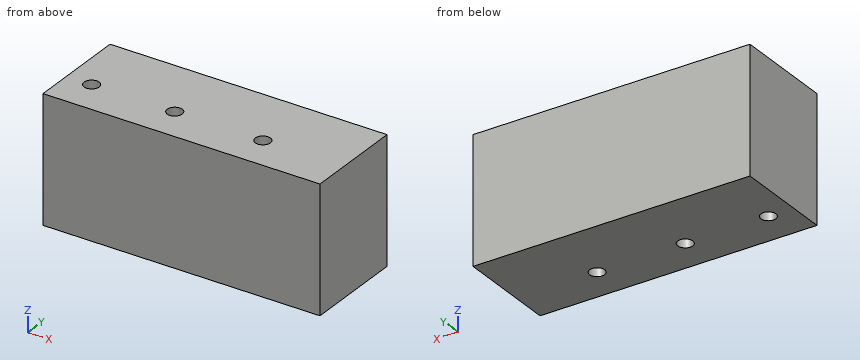
```python
from build123d import *

# Parameters (mm, degrees)
F0_W     = 55
F0_H     = 20
F1_DEPTH = 25
F2_R     = 1.5
F3_DEPTH = 25.001
F4_R     = 1.5
F5_DEPTH = 25.001
F6_R     = 1.5
F7_DEPTH = 25.001


with BuildPart() as f1:
    # F0 (on Top) → F1 (new body)
    with BuildSketch(Plane.XY):
        Rectangle(F0_W, F0_H)
    extrude(amount=F1_DEPTH)

    # F2 (on face) → F3 (cut, through all)
    with BuildSketch(Plane.XY.offset(25)):
        with Locations((-22.5, -3)):
            Circle(F2_R)
    extrude(amount=-F3_DEPTH, mode=Mode.SUBTRACT)

    # F4 (on face) → F5 (cut, through all)
    with BuildSketch(Plane.XY.offset(25)):
        with Locations((-6, -3)):
            Circle(F4_R)
    extrude(amount=-F5_DEPTH, mode=Mode.SUBTRACT)

    # F6 (on face) → F7 (cut, through all)
    with BuildSketch(Plane.XY.offset(25)):
        with Locations((11.5, -3)):
            Circle(F6_R)
    extrude(amount=-F7_DEPTH, mode=Mode.SUBTRACT)


solid = f1.part
```
For this review, take the finished solid that the model builds, in its own axes (mm). Give positions to 0.01 mm unless a question says otherwise; leave off trailing zeros. Order: outer loops, then holes, each group sorted by start corner. A loop starts at its lowest first (then second) coordinate and runs counter-clockwise, first axis right, second up.
1) Take a section at C-C (z = 8.75). Give the boundary of the cut face in (x, y), then the cut area to 3 significant figures.
2) Take a section at A-A (x = -22.5). Give the boundary of the cut face in (y, z).
3) Insertion check: pin 1 (1.8 mm diameter, centred on x = -6, y = -3, fed in from +Z). The pin has a flat end and moves straight along its axis. Give the tip position at first contact, or say it passes through.
4) Wall thickness on line 1 (X direction, y = -2.5, z = 15); line 2 (Y direction, x = -6, z = 7.5); line 3 (X direction, y = -2.25, z = 13.25): over which ranges is each line inside the solid? List them lowest first.
5) Take a section at B-B (y = -3). Give the boundary of the cut face in (x, z).
Derived:
1. outline: (-27.5, -10) - (27.5, -10) - (27.5, 10) - (-27.5, 10) - close; hole circle Ø3 at (-22.5, -3); hole circle Ø3 at (-6, -3); hole circle Ø3 at (11.5, -3)
1. area: 1,080 mm2
2. outline: (-10, 0) - (-4.5, 0) - (-4.5, 25) - (-10, 25) - close; (-1.5, 0) - (10, 0) - (10, 25) - (-1.5, 25) - close
3. pin 1: passes through
4. line 1: x = -27.5 to -23.91, -21.09 to -7.41, -4.59 to 10.09, 12.91 to 27.5
4. line 2: y = -10 to -4.5, -1.5 to 10
4. line 3: x = -27.5 to -23.8, -21.2 to -7.3, -4.7 to 10.2, 12.8 to 27.5
5. outline: (-27.5, 0) - (-24, 0) - (-24, 25) - (-27.5, 25) - close; (-21, 0) - (-7.5, 0) - (-7.5, 25) - (-21, 25) - close; (-4.5, 0) - (10, 0) - (10, 25) - (-4.5, 25) - close; (13, 0) - (27.5, 0) - (27.5, 25) - (13, 25) - close
